from build123d import *

# Parameters (mm, degrees)
F0_W     = 60
F0_H     = 60
F0_R     = 2.25
F0_R_2   = 19.05
F0_R_3   = 4
F1_DEPTH = 100
F2_DEPTH = 24.5
F4_DEPTH = 20
F5_DEPTH = 1.6
F6_DEPTH = 25
F7_R     = 3.5321510556
F8_DEPTH = 5


with BuildPart() as f1:
    # F0 (on Front) → F1 (new body)
    with BuildSketch(Plane.XZ):
        Rectangle(F0_W, F0_H)
        with Locations((-23.65, -23.65)):
            Circle(F0_R, mode=Mode.SUBTRACT)
        with Locations((23.65, -23.65)):
            Circle(F0_R, mode=Mode.SUBTRACT)
        with Locations((-23.65, 23.65)):
            Circle(F0_R, mode=Mode.SUBTRACT)
        Circle(F0_R_2, mode=Mode.SUBTRACT)
        with Locations((23.65, 23.65)):
            Circle(F0_R, mode=Mode.SUBTRACT)
        Circle(F0_R_2)
        Circle(F0_R_3, mode=Mode.SUBTRACT)
        Circle(F0_R_3)
        with Locations((-23.65, 23.65)):
            Circle(F0_R)
        with Locations((23.65, 23.65)):
            Circle(F0_R)
        with Locations((23.65, -23.65)):
            Circle(F0_R)
        with Locations((-23.65, -23.65)):
            Circle(F0_R)
    extrude(amount=-F1_DEPTH)

    # F0 (on Front) → F2 (join)
    with BuildSketch(Plane.XZ):
        Circle(F0_R_3)
    extrude(amount=F2_DEPTH)

    # F3 (on face) → F4 (cut)
    with BuildSketch(Plane.XZ.offset(24.5)):
        with BuildLine():
            ThreePointArc((1.9364916731, 3.5), (0, 4), (-1.9364916731, 3.5))
            Line((-1.9364916731, 3.5), (1.9364916731, 3.5))
        make_face()
    extrude(amount=-F4_DEPTH, mode=Mode.SUBTRACT)

    # F0 (on Front) → F5 (join)
    with BuildSketch(Plane.XZ):
        Circle(F0_R_2)
        Circle(F0_R_3, mode=Mode.SUBTRACT)
    extrude(amount=F5_DEPTH)

    # F0 (on Front) → F6 (cut)
    with BuildSketch(Plane.XZ):
        with Locations((-23.65, 23.65)):
            Circle(F0_R)
        with Locations((23.65, 23.65)):
            Circle(F0_R)
        with Locations((23.65, -23.65)):
            Circle(F0_R)
        with Locations((-23.65, -23.65)):
            Circle(F0_R)
    extrude(amount=-F6_DEPTH, mode=Mode.SUBTRACT)

    # F7 (on face) → F8 (join)
    with BuildSketch(Plane.XY.offset(30)):
        with Locations((0, 92.517465353)):
            Circle(F7_R)
    extrude(amount=F8_DEPTH)


solid = f1.part
Read the model definition and answer for the solid it produces. Units are mm, in the model's axes. A direction names the side the tool comes from. Coordinates: 2 decimals unless noted, no trailing zeros. Write each loop counter-clockwise with the first axis right and the second up, starting at its lowest first coordinate (ties: lowest second). Pieces come first, ordered by that corner, then holes. Notation, with made-up numbers: M 55.5,-25 L 102.5,-25 A28 ccw 102.5,11 Z; hole C -5.5,-25 d5. An arc over 180 degrees is marked long. Use a Markdown table: item, result.
Q1. The part is cut by section B-B, the plane z = 23.65. Write down the section's boundary in (x, y), then the cut area to 4 significant figures.
Answer block:
| item | result |
|---|---|
| outline | M -30,0 L -25.9,0 L -25.9,25 L -21.4,25 L -21.4,0 L 21.4,0 L 21.4,25 L 25.9,25 L 25.9,0 L 30,0 L 30,100 L -30,100 Z |
| area | 5,775 mm2 |
Q2. The part is cut by section A-A, the plane x = 0. Write down the section's boundary in (y, z), then the cut area to 3 significant figures.
Answer block:
| item | result |
|---|---|
| outline | M -24.5,-4 L -1.6,-4 L -1.6,-19.05 L 0,-19.05 L 0,-30 L 100,-30 L 100,30 L 96.05,30 L 96.05,35 L 88.99,35 L 88.99,30 L 0,30 L 0,19.05 L -1.6,19.05 L -1.6,4 L -4.5,4 L -4.5,3.5 L -24.5,3.5 Z |
| area | 6,270 mm2 |
Q3. The part is cut by section D-D, the plane x = -23.65. Write down the section's boundary in (y, z), then the cut area to 4 significant figures.
Answer block:
| item | result |
|---|---|
| outline | M 0,-30 L 100,-30 L 100,30 L 0,30 L 0,25.9 L 25,25.9 L 25,21.4 L 0,21.4 L 0,-21.4 L 25,-21.4 L 25,-25.9 L 0,-25.9 Z |
| area | 5,775 mm2 |
Q4. Determine the mould class of faces 6 (the face through (0, 49, -30)), 7 (the face through (-30, 49, 0)), 8 (the face through (-24, 25, 24)) for opening direction X: released by +X, released by -X, zero draft, split by the parting line, or undercut.
Answer block:
| item | result |
|---|---|
| face 6 | zero draft |
| face 7 | released by -X |
| face 8 | undercut |
Q5. Which of the six approach directions +Z, -Z, +X, -X, +Y, -Y give full straight-line access (tool end or side, diameter ignored) to faces 1 (the face through (0, -15, 3.5)), 2 (the face through (0, -24.5, 0)), 3 (the face through (24.86, 12.325, 25.547)), 4 (the face through (0, 93, 35)), 5 (the face through (-0.77, 89.07, 32.47))?
Answer block:
| item | result |
|---|---|
| face 1 | +Z, +X, -X, -Y |
| face 2 | +Z, -Z, +X, -X, -Y |
| face 3 | -Y |
| face 4 | +Z, +X, -X, +Y, -Y |
| face 5 | +Z |
Q6. Each of these flat-tipped pins is pushed along its axis until it touches: pin 1 Ø2 at (x, z) = (-23, -23) entering from -Y; pin 2 Ø6 at (x, z) = (-4.5, 3.5) entering from -Y; pin 3 Ø12 at (x, z) = (11, 1) entering from -Y; pin 4 Ø7 at (x, z) = (-23.65, -23.65) entering from -Y. Where does it stop, or does it pass through?
Answer block:
| item | result |
|---|---|
| pin 1 | stops at y = 25 |
| pin 2 | stops at y = -24.5 |
| pin 3 | stops at y = -1.6 |
| pin 4 | stops at y = 0 |
Q7. The part is cut by section C-C, the plane y = 44.5. Write down the section's boundary in (x, z), then the cut area to 3 significant figures.
Answer block:
| item | result |
|---|---|
| outline | M -30,-30 L 30,-30 L 30,30 L -30,30 Z |
| area | 3,600 mm2 |
Q8. Straight lines are drawn through the part: L1, parallel to Z at x = 23.65, y = 9.5; L2, parallel to X at y = 19, z = 23; L3, parallel to Y at x = 26.5, z = 24.5. For each, find the intervals that lie inside material, in ascending order. Write a range as [from, to].
Answer block:
| item | result |
|---|---|
| L1 | z = [-30, -25.9], [-21.4, 21.4], [25.9, 30] |
| L2 | x = [-30, -25.8], [-21.5, 21.5], [25.8, 30] |
| L3 | y = [0, 100] |
